Work out the finished part from the listing and answer in its coordinate system (mm). Face numbers are marked on the shaded views. Coordinates: 2 decimals unless noted, no trailing zeros. Loops run counter-clockwise (first coordinate to the right, second up) from the corner with the lowest first, then second, coordinate; pieces in that order, holes last. Notation, with made-up numbers: (67.5, -10) -> (117.5, -10) arc R19 ccw to (117.5, 18) -> close; hole circle Ø6 at (45, 5.5). An arc over 180 degrees is marked (long way). Use a Markdown table: item, result. Add a question column.
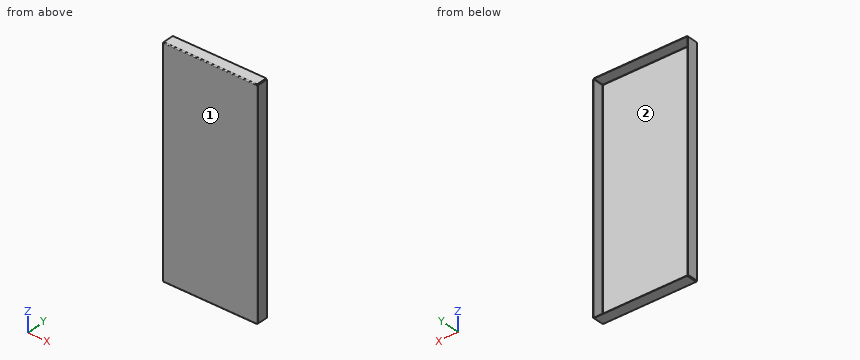
Autodesk Inventor part; units mm, degrees
ref_plane "YZ Plane" through (0, 0, 0) normal (1, 0, 0) x (0, 1, 0)
ref_plane "XZ Plane" through (0, 0, 0) normal (0, 1, 0) x (-1, 0, 0)
ref_plane "XY Plane" through (0, 0, 0) normal (0, 0, 1) x (1, 0, 0)
sketch "Sketch1" plane through (0, 0, 0) normal (0, 1, 0) x (-1, 0, 0)
  line L0 (72.3629, 154.3951) -> (-92.6371, 154.3951)
  line L1 (-92.6371, 154.3951) -> (-92.6371, -230.4049)
  line L2 (-92.6371, -230.4049) -> (72.3629, -230.4049)
  line L3 (72.3629, -230.4049) -> (72.3629, 154.3951)
  point P0 (0, 0)
  dimension "d0" = 165
  dimension "d1" = 384.8
extrude "Plate1" add sketch "Sketch1" along normal blind 0.8
sketch "Sketch2" plane through (92.6371, 0, 153.5951) normal (0, 0, 1) x (1, 0, 0)
  line L0 (-165, 0) -> (0, 0)
  line L1 (0, 0) -> (0, 20)
  line L2 (0, 20) -> (-165, 20)
  line L3 (-165, 20) -> (-165, 0)
edge flange "Flange1" height 20 angle 90 thickness 0.8 bend radius 0.8 thickness toward (0, 0, 1) relief tear relief width 0.8 relief depth 0.4 corner gap 0.8 corner form 2 edges at (10.1371, 0.8, 154.3951) (-72.3629, 0.8, -38.0049) (92.6371, 0.8, -38.0049) (10.1371, 0.8, -230.4049) wall of the first edge with corners at (-72.3629, 0, 153.5951) (92.6371, 0, 153.5951) (92.6371, 20, 153.5951) (-72.3629, 20, 153.5951)
bend "Bend1"
corner "Corner1"
equation "\"d2\" = Thickness"
equation "\"d3\" = BendReliefWidth"
equation "\"d4\" = BendReliefDepth"
equation "\"d5\" = MinimumRemnant"
equation "\"d6\" = TransitionRadius"
equation "\"d9\" = BendRadius"
equation "\"d10\" = CornerReliefSize"
equation "\"d11\" = GapSize"
equation "\"d12\" = JacobiRadiusSize"
equation "\"BendRadius\" = Thickness"
equation "\"BendReliefWidth\" = Thickness"
equation "\"BendReliefDepth\" = 0.5 * Thickness"
equation "\"CornerReliefSize\" = 4 * Thickness"
equation "\"MinimumRemnant\" = 2 * Thickness"
equation "\"TransitionRadius\" = BendRadius"
equation "\"JacobiRadiusSize\" = BendRadius"
equation "\"GapSize\" = Thickness"
properties part number "Back_plate"
Item 1: For a pull along Z with two mould halves and no side action, classify the marked faces 1 and 2 as +Z half, -Z half, draft (parallel to the pull), parting line (faces both ways), or undercut.
Item 2: Section A-A (y = 7) is taken. Determine the outline of the cut face in (x, z), then the cut area to 3 significant figures.
Item 3: Section C-C (x = 18) is taken. Determine the outline of the cut face in (y, z), then the cut area to 3 significant figures.
Item 4: Given pin 1 (0.8 mm diameter, centred on x = -71, y = 1, fed in from -Z); pin 2 (0.9 mm diameter, centred on x = -72, y = 12.5, fed in from +Z); pin 3 (0.5 mm diameter, centred on x = 92, y = 1, fed in from +Z), each flat-ended and moving along its own axis, determine where each tip first touches the part or whether it passes through.
Item 5: Find the intervals of material crossed by probe 1 along Z at (x, y) = (7, 6.75); probe 2 along X at (y, z) = (9.5, 60); probe 3 along Y at (x, z) = (-21, -144), in increasing order.
Item 6: Section B-B (z = 74.5) is taken. Determine the outline of the cut face in (x, y).
Output:
| question | item | result |
|---|---|---|
| 1 | face 1 | draft |
| 1 | face 2 | undercut |
| 2 | outline | (-72.36, -229.04) -> (-71.56, -229.04) -> (-71.56, 153.03) -> (-72.36, 153.03) -> close; (-71, -230.4) -> (91.27, -230.4) -> (91.27, -229.6) -> (-71, -229.6) -> close; (-71, 153.6) -> (91.27, 153.6) -> (91.27, 154.4) -> (-71, 154.4) -> close; (91.84, -229.04) -> (92.64, -229.04) -> (92.64, 153.03) -> (91.84, 153.03) -> close |
| 2 | area | 871 mm2 |
| 3 | outline | (0, -228.8) arc R1.6 ccw to (1.6, -230.4) -> (20, -230.4) -> (20, -229.6) -> (1.6, -229.6) arc R0.8 cw to (0.8, -228.8) -> (0.8, 152.8) arc R0.8 cw to (1.6, 153.6) -> (20, 153.6) -> (20, 154.4) -> (1.6, 154.4) arc R1.6 ccw to (0, 152.8) -> close |
| 3 | area | 338 mm2 |
| 4 | pin 1 | stops at z = -230.38 |
| 4 | pin 2 | stops at z = 153.03 |
| 4 | pin 3 | stops at z = 152.8 |
| 5 | probe 1 | z = -230.4 to -229.6, 153.6 to 154.4 |
| 5 | probe 2 | x = -72.36 to -71.56, 91.84 to 92.64 |
| 5 | probe 3 | y = 0 to 0.8 |
| 6 | outline | (-72.36, 1.6) arc R1.6 ccw to (-70.76, 0) -> (91.04, 0) arc R1.6 ccw to (92.64, 1.6) -> (92.64, 20) -> (91.84, 20) -> (91.84, 1.6) arc R0.8 cw to (91.04, 0.8) -> (-70.76, 0.8) arc R0.8 cw to (-71.56, 1.6) -> (-71.56, 20) -> (-72.36, 20) -> close |
